Read the model definition and answer for the solid it produces. Units are mm, in the model's axes. A direction names the side the tool comes from. Coordinates: 2 decimals unless noted, no trailing zeros. Order: outer loops, then holes, each group sorted by start corner. A loop starts at its lowest first (then second) coordinate and runs counter-clockwise, first axis right, second up. Notation, with made-up numbers: M 0.25,-14.5 L 21.25,-14.5 A20 ccw 21.25,8.5 Z; hole C 59.5,41 d9. An arc over 180 degrees is marked long. One line per question, with ' | ' between items. Start each with the question number.
1) Consider probe 1 along X at (y, z) = (28.5, 2.3); probe 2 along X at (y, z) = (19.5, 0.95); probe 3 along Z at (x, y) = (34.5, 17.75). Determine where each line is inside the solid, lowest interval first.
2) A tool of negligible diameter and unlimited length cuts with its end or side. For faces 4 (the face through (24.43, 40.4, 2.46)), 5 (the face through (-37, 15, 2)), 6 (the face through (-33, 30, 2)), 7 (the face through (33, 30, 2)), from which of +Z, -Z, +X, -X, +Y, -Y can it reach the whole face along a straight path? Write none if from no direction.
3) The mould has two halves that part along X. Classify faces 1 (the face through (25, 20, 2)), 2 (the face through (29, 35, 2)), 3 (the face through (8, 43, 0)): +X half, -X half, draft (parallel to the pull), parting line (faces both ways), or undercut.
4) Find section D-D, the plane x = 19. Write down the section's boundary in (y, z), plus the area to 3 significant figures.
5) Given P1, Ø3, axis at x = 14.5, z = 0.5, coming from the -Y side; P2, Ø2.5, axis at x = 35, z = 3.5, coming from the +Y side; P3, Ø2.5, axis at y = 33, z = 2, coming from the +X side; P4, Ø2, axis at x = 34.5, z = 2.5, coming from the +Y side, each flat-ended and moving along its own axis, determine where each tip first touches the part or whether it passes through.
6) Find section B-B, the plane x = 34.5. Write down the section's boundary in (y, z).
7) Find section A-A, the plane y = 20. Write down the section's boundary in (x, z).
8) Find section C-C, the plane z = 2.5. Write down the section's boundary in (x, y), plus the area to 3 significant figures.
from build123d import *

# Parameters (mm, degrees)
PAD_DEPTH    = 5
SKETCH001_R  = 1.25
POCKET_DEPTH = 30.001


with BuildPart() as part:
    # Sketch → Pad (new body)
    with BuildSketch(Plane.XY):
        with BuildLine():
            Line((0, 41), (23, 41))
            ThreePointArc((25, 39), (24.414214, 40.414214), (23, 41))
            Line((25, 39), (25, 0))
            Line((25, 0), (37, 0))
            Line((37, 30), (37, 0))
            Line((29, 30), (37, 30))
            Line((29, 39), (29, 30))
            ThreePointArc((29, 39), (27.242641, 43.242641), (23, 45))
            Line((0, 45), (23, 45))
            Line((0, 45), (0, 41))
        make_face()
    extrude(amount=PAD_DEPTH)

    # Sketch001 (on Face7 of Pad) → Pocket (cut, through all)
    with BuildSketch(Plane(origin=(0, 30, 0), x_dir=(-1, 0, 0), z_dir=(0, 1, 0))):
        with Locations((-34.5, 2.5)):
            Circle(SKETCH001_R)
    extrude(amount=-POCKET_DEPTH, mode=Mode.SUBTRACT)

    # Mirrored: part across YZ


with BuildPart() as part_1:
    add(part.part)
    add(part.part.mirror(Plane.YZ))


solid = part_1.part
Report:
1) probe 1: x = -37 to -35.73, -33.27 to -25, 25 to 33.27, 35.73 to 37 | probe 2: x = -37 to -25, 25 to 37 | probe 3: z = 0 to 1.25, 3.75 to 5
2) face 4: +Z, -Z, -Y | face 5: +Z, -Z, -X, +Y, -Y | face 6: +Z, -Z, -X, +Y | face 7: +Z, -Z, +X, +Y
3) face 1: undercut | face 2: +X half | face 3: draft
4) outline: M 41,0 L 45,0 L 45,5 L 41,5 Z | area: 20.0 mm^2
5) P1: stops at y = 41 | P2: stops at y = 30 | P3: stops at x = 29 | P4: passes through
6) outline: M 0,0 L 30,0 L 30,1.25 L 0,1.25 Z; M 0,3.75 L 30,3.75 L 30,5 L 0,5 Z
7) outline: M -37,0 L -25,0 L -25,5 L -37,5 Z; M 25,0 L 37,0 L 37,5 L 25,5 Z; hole C -34.5,2.5 d2.5; hole C 34.5,2.5 d2.5
8) outline: M -37,0 L -35.75,0 L -35.75,30 L -37,30 Z; M -33.25,0 L -25,0 L -25,39 A2 cw -23,41 L 23,41 A2 cw 25,39 L 25,0 L 33.25,0 L 33.25,30 L 29,30 L 29,39 A6 ccw 23,45 L -23,45 A6 ccw -29,39 L -29,30 L -33.25,30 Z; M 35.75,0 L 37,0 L 37,30 L 35.75,30 Z | area: 876 mm^2
